from build123d import *

# Parameters (mm, degrees)
BOSS_EXTRUDE1_DEPTH = 1.25
SKETCH2_W           = 1
SKETCH2_H           = 0.325
BOSS_EXTRUDE2_DEPTH = 2
SKETCH3_W           = 1
SKETCH3_H           = 0.325
BOSS_EXTRUDE3_DEPTH = 2


with BuildPart() as part:
    # Sketch1 → Boss-Extrude1 (new body)
    with BuildSketch(Plane.XY):
        Polygon((1, 0), (9, 0), (9, -0.325), (10, -0.325), (10, -1), (17, -1), (17, 1), (10, 1), (0, 1), (-7, 1), (-7, -1), (0, -1), (0, -0.325), (1, -0.325), align=None)
    extrude(amount=BOSS_EXTRUDE1_DEPTH)

    # Sketch2 → Boss-Extrude2 (add)
    with BuildSketch(Plane.XY.offset(1.25)):
        with Locations((0.5, -0.1625)):
            Rectangle(SKETCH2_W, SKETCH2_H)
        with Locations((9.5, -0.1625)):
            Rectangle(SKETCH2_W, SKETCH2_H)
    extrude(amount=BOSS_EXTRUDE2_DEPTH)

    # Sketch3 → Boss-Extrude3 (add)
    with BuildSketch(Plane(origin=(0, 0, 0), x_dir=(-1, 0, 0), z_dir=(0, 0, -1))):
        with Locations((-9.5, -0.1625)):
            Rectangle(SKETCH3_W, SKETCH3_H)
        with Locations((-0.5, -0.1625)):
            Rectangle(SKETCH3_W, SKETCH3_H)
    extrude(amount=BOSS_EXTRUDE3_DEPTH)


solid = part.part
Input: part model. Units: mm. Frame: model coordinates. A direction names the side the tool comes from. Give positions to 0.01 mm unless a question says otherwise; leave off trailing zeros. Order: outer loops, then holes, each group sorted by start corner. A loop starts at its lowest first (then second) coordinate and runs counter-clockwise, first axis right, second up.
Q1. Draft query along X for faces 5 (the flat face through (0.5, -0.325, 0.7)), 6 (the flat face through (-7, 0, 1)), 7 (the flat face through (-4, -1, 1)). Return one class per face: +X half, -X half, draft (parallel to the pull), parting line (faces both ways), or undercut.
Checked values:
face 5: undercut
face 6: -X half
face 7: draft
Q2. Section C-C on x = 9.5. Output: boundary loops of the cut face in (y, z) (3 decimals).
Checked values:
outline: (-0.325, -2) - (0, -2) - (0, 0) - (1, 0) - (1, 1.25) - (0, 1.25) - (0, 3.25) - (-0.325, 3.25) - close
Q3. Ray query, probe 1 along Z at (x, y) = (15.75, -0.85); probe 2 along Y at (x, z) = (4.25, 0.35); probe 3 along Y at (x, z) = (9.5, 2.4) (3 decimals). Return the intervals inside material, ascending.
Checked values:
probe 1: z = 0 to 1.25
probe 2: y = 0 to 1
probe 3: y = -0.325 to 0
Q4. Section D-D on y = 0.65. Output: boundary loops of the cut face in (x, z), and give its area (3 significant figures).
Checked values:
outline: (-7, 0) - (17, 0) - (17, 1.25) - (-7, 1.25) - close
area: 30.0 mm2
Q5. Contact query for flat-ended pins moving along their axis: pin 1 Ø0.8 at (x, z) = (9.5, 1) entering from -Y (3 decimals); pin 2 Ø0.5 at (x, z) = (9.5, -1) entering from +Y; pin 3 Ø1 at (x, z) = (7, 1) entering from -Y. Output: stop coordinate, or through.
Checked values:
pin 1: stops at y = -0.325
pin 2: stops at y = 0
pin 3: stops at y = 0
Q6. Section A-A on y = -0.8. Output: boundary loops of the cut face in (x, z).
Checked values:
outline: (-7, 0) - (0, 0) - (0, 1.25) - (-7, 1.25) - close; (10, 0) - (17, 0) - (17, 1.25) - (10, 1.25) - close
Q7. Section B-B on z = -0.65. Output: boundary loops of the cut face in (x, y) (3 decimals).
Checked values:
outline: (0, -0.325) - (1, -0.325) - (1, 0) - (0, 0) - close; (9, -0.325) - (10, -0.325) - (10, 0) - (9, 0) - close
Q8. Set-up query: faces 1 (the flat face through (9.5, 0, -1)), 2 (the flat face through (17, 0, 1)), 3 (the flat face through (9.5, -0.325, 0.7)), 4 (the flat face through (0.5, 0, 2.2)). Return all of +Z, -Z, +X, -X, +Y, -Y with unobstructed straight access to the full face (end or side cutting, diameter ignored); none if empty.
Checked values:
face 1: -Z, +X, -X, +Y
face 2: +Z, -Z, +X, +Y, -Y
face 3: +Z, -Z, -Y
face 4: +Z, +X, -X, +Y
